from build123d import *

# Parameters (mm, degrees)
EXTRUDE_1_DEPTH     = 5
CUT_EXTRUDE_1_REACH = 61.055
SKETCH_2_R          = 3.5
SKETCH_2_R_2        = 7.5
SKETCH_2_R_3        = 1.65


with BuildPart() as part:
    # 草图1 → 凸台-拉伸1 (new body)
    with BuildSketch(Plane(origin=(0, 0, 0), x_dir=(1, 0, 0), z_dir=(0, 1, 0))):
        with BuildLine():
            Line((45, -12.5), (-45, -12.5))
            ThreePointArc((-45, -12.5), (-57.5, 0), (-45, 12.5))
            Line((-45, 12.5), (45, 12.5))
            ThreePointArc((45, 12.5), (57.5, 0), (45, -12.5))
        make_face()
    extrude(amount=EXTRUDE_1_DEPTH)

    # 草图2 → 切除-拉伸1 (cut, up to next)
    with BuildSketch(Plane(origin=(0, 5, 0), x_dir=(1, 0, 0), z_dir=(0, 1, 0)), mode=Mode.PRIVATE) as cut_extrude_1_sk1:
        with Locations(Location((-45, 0, 0), (0, 0, 270))):
            Circle(SKETCH_2_R)
    cut_extrude_1_tool1 = extrude(cut_extrude_1_sk1.sketch, amount=-CUT_EXTRUDE_1_REACH, mode=Mode.PRIVATE) & part.part
    # 草图2 → 切除-拉伸1 (cut, up to next)
    with BuildSketch(Plane(origin=(0, 5, 0), x_dir=(1, 0, 0), z_dir=(0, 1, 0)), mode=Mode.PRIVATE) as cut_extrude_1_sk2:
        with Locations(Location((45, 0, 0), (0, 0, 270))):
            Circle(SKETCH_2_R_2)
    cut_extrude_1_tool2 = extrude(cut_extrude_1_sk2.sketch, amount=-CUT_EXTRUDE_1_REACH, mode=Mode.PRIVATE) & part.part
    # 草图2 → 切除-拉伸1 (cut, up to next)
    with BuildSketch(Plane(origin=(0, 5, 0), x_dir=(1, 0, 0), z_dir=(0, 1, 0)), mode=Mode.PRIVATE) as cut_extrude_1_sk3:
        with Locations(Location((-45, 7, 0), (0, 0, 270))):
            Circle(SKETCH_2_R_3)
    cut_extrude_1_tool3 = extrude(cut_extrude_1_sk3.sketch, amount=-CUT_EXTRUDE_1_REACH, mode=Mode.PRIVATE) & part.part
    # 草图2 → 切除-拉伸1 (cut, up to next)
    with BuildSketch(Plane(origin=(0, 5, 0), x_dir=(1, 0, 0), z_dir=(0, 1, 0)), mode=Mode.PRIVATE) as cut_extrude_1_sk4:
        with Locations(Location((-38, 0, 0), (0, 0, 270))):
            Circle(SKETCH_2_R_3)
    cut_extrude_1_tool4 = extrude(cut_extrude_1_sk4.sketch, amount=-CUT_EXTRUDE_1_REACH, mode=Mode.PRIVATE) & part.part
    # 草图2 → 切除-拉伸1 (cut, up to next)
    with BuildSketch(Plane(origin=(0, 5, 0), x_dir=(1, 0, 0), z_dir=(0, 1, 0)), mode=Mode.PRIVATE) as cut_extrude_1_sk5:
        with Locations(Location((-45, -7, 0), (0, 0, 270))):
            Circle(SKETCH_2_R_3)
    cut_extrude_1_tool5 = extrude(cut_extrude_1_sk5.sketch, amount=-CUT_EXTRUDE_1_REACH, mode=Mode.PRIVATE) & part.part
    # 草图2 → 切除-拉伸1 (cut, up to next)
    with BuildSketch(Plane(origin=(0, 5, 0), x_dir=(1, 0, 0), z_dir=(0, 1, 0)), mode=Mode.PRIVATE) as cut_extrude_1_sk6:
        with Locations(Location((-52, 0, 0), (0, 0, 270))):
            Circle(SKETCH_2_R_3)
    cut_extrude_1_tool6 = extrude(cut_extrude_1_sk6.sketch, amount=-CUT_EXTRUDE_1_REACH, mode=Mode.PRIVATE) & part.part
    add(cut_extrude_1_tool1.solids().sort_by_distance((-45, 5, 0))[0], mode=Mode.SUBTRACT)
    add(cut_extrude_1_tool2.solids().sort_by_distance((45, 5, 0))[0], mode=Mode.SUBTRACT)
    add(cut_extrude_1_tool3.solids().sort_by_distance((-45, 5, -7))[0], mode=Mode.SUBTRACT)
    add(cut_extrude_1_tool4.solids().sort_by_distance((-38, 5, 0))[0], mode=Mode.SUBTRACT)
    add(cut_extrude_1_tool5.solids().sort_by_distance((-45, 5, 7))[0], mode=Mode.SUBTRACT)
    add(cut_extrude_1_tool6.solids().sort_by_distance((-52, 5, 0))[0], mode=Mode.SUBTRACT)


solid = part.part
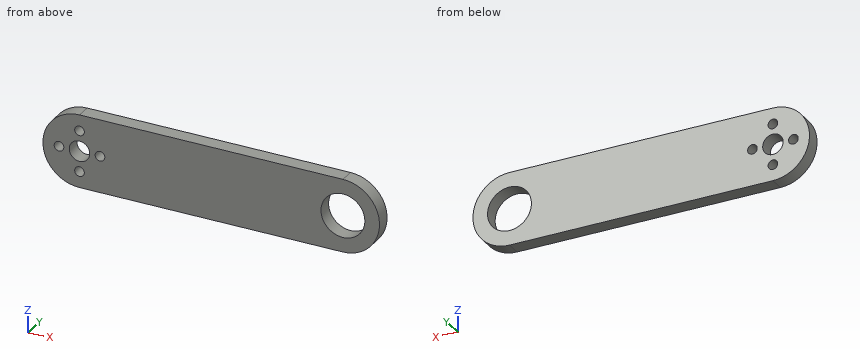
Geometry check sheet. Reference: the model listing, model coordinates, mm. Give positions to 0.01 mm unless a question says otherwise; leave off trailing zeros. Loops run counter-clockwise (first coordinate to the right, second up) from the corner with the lowest first, then second, coordinate; pieces in that order, holes last.
(1) Section check C-C on y = 3.1. Record the cut outline in (x, z), then the cut area to 3 significant figures.
From the geometry:
outline: (-45, -12.5) - (45, -12.5) arc R12.5 ccw to (45, 12.5) - (-45, 12.5) arc R12.5 ccw to start; hole circle Ø3.3 at (-52, 0); hole circle Ø7 at (-45, 0); hole circle Ø3.3 at (-45, -7); hole circle Ø3.3 at (-45, 7); hole circle Ø3.3 at (-38, 0); hole circle Ø15 at (45, 0)
area: 2,490 mm2
(2) Depth check by flat-ended pin: pin 1 Ø3 at (y, z) = (1, -4.5) entering from +X; pin 2 Ø13.5 at (x, z) = (45, 0) entering from -Y. Enter the tip coordinate at first touch or a pass-through.
From the geometry:
pin 1: stops at x = 57.13
pin 2: passes through
(3) Section check D-D on x = -52. Record the cut outline in (y, z).
From the geometry:
outline: (0, -10.36) - (5, -10.36) - (5, -1.65) - (0, -1.65) - close; (0, 1.65) - (5, 1.65) - (5, 10.36) - (0, 10.36) - close
(4) Section check B-B on x = -38. Record the cut outline in (y, z).
From the geometry:
outline: (0, -12.5) - (5, -12.5) - (5, -1.65) - (0, -1.65) - close; (0, 1.65) - (5, 1.65) - (5, 12.5) - (0, 12.5) - close
(5) Section check A-A on z = 0. Record the cut outline in (x, y).
From the geometry:
outline: (-57.5, 0) - (-53.65, 0) - (-53.65, 5) - (-57.5, 5) - close; (-50.35, 0) - (-48.5, 0) - (-48.5, 5) - (-50.35, 5) - close; (-41.5, 0) - (-39.65, 0) - (-39.65, 5) - (-41.5, 5) - close; (-36.35, 0) - (37.5, 0) - (37.5, 5) - (-36.35, 5) - close; (52.5, 0) - (57.5, 0) - (57.5, 5) - (52.5, 5) - close
(6) Thickness scan on L1, parallel to X at y = 3.2, z = 0; L2, parallel to X at y = 4.7, z = -6.25; L3, parallel to X at y = 2.5, z = -6.5. Record the ranges inside material, lowest first.
From the geometry:
L1: x = -57.5 to -53.65, -50.35 to -48.5, -41.5 to -39.65, -36.35 to 37.5, 52.5 to 57.5
L2: x = -55.83 to -46.47, -43.53 to 40.85, 49.15 to 55.83
L3: x = -55.68 to -46.57, -43.43 to 41.26, 48.74 to 55.68
